```python
from build123d import *

# Parameters (mm, degrees)
BOSS_EXTRUDE1_DEPTH          = 45
SKETCH2_W                    = 42
SKETCH2_H                    = 46.212418486
CUT_EXTRUDE1_DEPTH           = 23
SKETCH3_W                    = 39
SKETCH3_H                    = 1.5
BOSS_EXTRUDE2_DEPTH          = 2
SKETCH4_W                    = 39
SKETCH4_H                    = 1.5
BOSS_EXTRUDE3_DEPTH          = 3.5
SKETCH5_W                    = 39
SKETCH5_H                    = 1.5
BOSS_EXTRUDE4_DEPTH          = 2
SKETCH6_W                    = 39
SKETCH6_H                    = 1.5
BOSS_EXTRUDE5_DEPTH          = 3.5
F_8_0_8_DIAMETER_HOLE1_D     = 8
F_8_0_8_DIAMETER_HOLE1_DEPTH = 1.5
F_8_0_8_DIAMETER_HOLE2_D     = 8
F_8_0_8_DIAMETER_HOLE2_DEPTH = 1.5
F_8_0_8_DIAMETER_HOLE3_D     = 8
F_8_0_8_DIAMETER_HOLE3_DEPTH = 1.5
FILLET1_R                    = 1.5
SKETCH13_R                   = 1
CUT_EXTRUDE2_DEPTH           = 2
SKETCH14_W                   = 11
SKETCH14_H                   = 8
CUT_EXTRUDE3_DEPTH           = 45
FILLET2_R                    = 0.5


with BuildPart() as part:
    # Sketch1 → Boss-Extrude1 (new body)
    with BuildSketch(Plane(origin=(22.5, 0, 0), x_dir=(0, 0, -1), z_dir=(1, 0, 0))):
        with BuildLine():
            Line((-11, 30), (-11, 0))
            ThreePointArc((-11, 0), (0, -11), (11, 0))
            Line((11, 0), (11, 30))
            Line((11, 30), (-11, 30))
        make_face()
    extrude(amount=-BOSS_EXTRUDE1_DEPTH)

    # Sketch2 → Cut-Extrude1 (cut, through all)
    with BuildSketch(Plane.XY.offset(11)):
        with Locations((0, 5.393790757)):
            Rectangle(SKETCH2_W, SKETCH2_H)
    extrude(amount=-CUT_EXTRUDE1_DEPTH, mode=Mode.SUBTRACT)

    # Sketch3 → Boss-Extrude2 (add)
    with BuildSketch(Plane(origin=(0, 0, -11), x_dir=(-1, 0, 0), z_dir=(0, 0, -1))):
        with Locations((0, 29.25)):
            Rectangle(SKETCH3_W, SKETCH3_H)
    extrude(amount=BOSS_EXTRUDE2_DEPTH)

    # Sketch4 → Boss-Extrude3 (add)
    with BuildSketch(Plane.XZ.offset(-28.5)):
        with Locations((0, -12.25)):
            Rectangle(SKETCH4_W, SKETCH4_H)
    extrude(amount=BOSS_EXTRUDE3_DEPTH)

    # Sketch5 → Boss-Extrude4 (add)
    with BuildSketch(Plane.XY.offset(11)):
        with Locations((0, 29.25)):
            Rectangle(SKETCH5_W, SKETCH5_H)
    extrude(amount=BOSS_EXTRUDE4_DEPTH)

    # Sketch6 → Boss-Extrude5 (add)
    with BuildSketch(Plane.XZ.offset(-28.5)):
        with Locations((0, 12.25)):
            Rectangle(SKETCH6_W, SKETCH6_H)
    extrude(amount=BOSS_EXTRUDE5_DEPTH)

    # Ø8.0 (8) Diameter Hole1
    with Locations(Plane(origin=(0, 28.5, 0), x_dir=(-1, 0, 0), z_dir=(0, -1, 0))):
        with Locations((0, 0)):
            Hole(F_8_0_8_DIAMETER_HOLE1_D / 2, depth=F_8_0_8_DIAMETER_HOLE1_DEPTH)

    # Ø8.0 (8) Diameter Hole2
    with Locations(Plane(origin=(-21, 0, 0), x_dir=(0, 0, -1), z_dir=(1, 0, 0))):
        with Locations((0, 0)):
            Hole(F_8_0_8_DIAMETER_HOLE2_D / 2, depth=F_8_0_8_DIAMETER_HOLE2_DEPTH)

    # Ø8.0 (8) Diameter Hole3
    with Locations(Plane.ZY.offset(-21)):
        with Locations((0, 0)):
            Hole(F_8_0_8_DIAMETER_HOLE3_D / 2, depth=F_8_0_8_DIAMETER_HOLE3_DEPTH)

    # Fillet1
    fillet1_edges = [part.edges().sort_by_distance(p)[0] for p in [
        (0, 30, -13),
        (-22.5, 30, 0),
        (22.5, 30, 0),
        (0, 30, 13),
    ]]
    fillet(fillet1_edges, radius=FILLET1_R)

    # Sketch13 → Cut-Extrude2 (cut)
    with BuildSketch(Plane(origin=(0, 30, 0), x_dir=(1, 0, 0), z_dir=(0, 1, 0))):
        with Locations((0, 8)):
            Circle(SKETCH13_R)
        with Locations((0, -8)):
            Circle(SKETCH13_R)
    extrude(amount=-CUT_EXTRUDE2_DEPTH, mode=Mode.SUBTRACT)

    # Sketch14 → Cut-Extrude3 (cut)
    with BuildSketch(Plane(origin=(22.5, 0, 0), x_dir=(0, 0, -1), z_dir=(1, 0, 0))):
        with Locations((0, 18)):
            Rectangle(SKETCH14_W, SKETCH14_H)
    extrude(amount=-CUT_EXTRUDE3_DEPTH, mode=Mode.SUBTRACT)

    # Fillet2
    fillet2_edges = [part.edges().sort_by_distance(p)[0] for p in [
        (-21.75, 14, 5.5),
        (21.75, 14, 5.5),
        (-21.75, 22, 5.5),
        (21.75, 22, 5.5),
        (-21.75, 22, -5.5),
        (21.75, 22, -5.5),
        (-21.75, 14, -5.5),
        (21.75, 14, -5.5),
    ]]
    fillet(fillet2_edges, radius=FILLET2_R)


solid = part.part
```
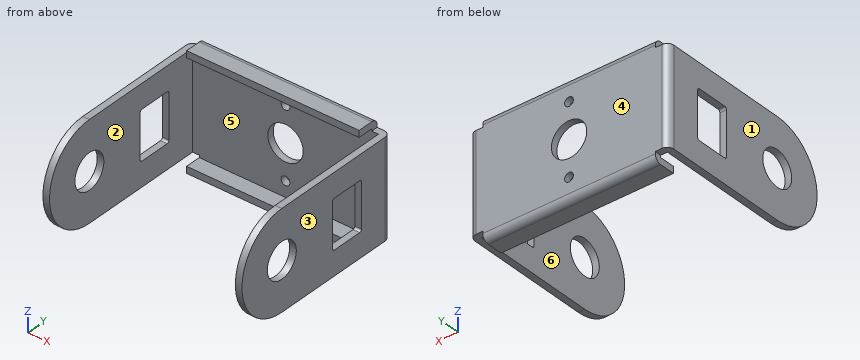
Geometry check sheet. Reference: the model listing, model coordinates, mm. Face numbers are marked on the shaded views. A direction names the side the tool comes from. Give positions to 0.01 mm unless a question says otherwise; leave off trailing zeros. Loops run counter-clockwise (first coordinate to the right, second up) from the corner with the lowest first, then second, coordinate; pieces in that order, holes last. Notation, with made-up numbers: M 88,65 L 96,65 A14 ccw 96,87 Z; hole C 16.5,-27.5 d11. An arc over 180 degrees is marked long. Write item = value, one per line.
(1) Sectioned sample at A-A, the plane y = 10.5. Record the cut outline in (x, z), plus the area to 3 significant figures.
Answer below:
outline = M -22.5,-11 L -21,-11 L -21,11 L -22.5,11 Z; M 21,-11 L 22.5,-11 L 22.5,11 L 21,11 Z
area = 66.0 mm2
(2) Sectioned sample at D-D, the plane y = 3. Record the cut outline in (x, z).
Answer below:
outline = M -22.5,-11 L -21,-11 L -21,-2.65 L -22.5,-2.65 Z; M -22.5,2.65 L -21,2.65 L -21,11 L -22.5,11 Z; M 21,-11 L 22.5,-11 L 22.5,-2.65 L 21,-2.65 Z; M 21,2.65 L 22.5,2.65 L 22.5,11 L 21,11 Z
(3) Sectioned sample at C-C, the plane z = 0. State how many separate pieces and enclosed holes the cut face has, plus the area to 3 significant figures.
Answer below:
separate_pieces = 6
enclosed_holes = 0
area = 125 mm2
(4) Gauge pin test, flat ends, axial feed: pin 1 Ø3.5 at (x, y) = (20.5, 11.5) entering from -Z; pin 2 Ø1.6 at (y, z) = (27, 12.5) entering from +X; pin 3 Ø11.5 at (x, z) = (-10, 4.5) entering from -Y; pin 4 Ø0.9 at (x, y) = (-20.5, 8) entering from -Z. Record the tip position at first contact, or that the pin passes through.
Answer below:
pin_1 = -11
pin_2 = 19.5
pin_3 = 28.5
pin_4 = through
(5) Tool access check on the marked faces 5 and 6. Record the directions out of +Z, -Z, +X, -X, +Y, -Y that give a thin tool (end or side, any length) a straight path to the whole face; none if there is none.
Answer below:
face_5 = -Y
face_6 = +Z, -Z, -Y
(6) Sectioned sample at B-B, the plane x = 0. Record the cut outline in (y, z).
Answer below:
outline = M 25,-13 L 28.5,-13 A1.5 ccw 30,-11.5 L 30,-9 L 28.5,-9 L 28.5,-11.5 L 25,-11.5 Z; M 25,11.5 L 28.5,11.5 L 28.5,9 L 30,9 L 30,11.5 A1.5 ccw 28.5,13 L 25,13 Z; M 28.5,-7 L 30,-7 L 30,-4 L 28.5,-4 Z; M 28.5,4 L 30,4 L 30,7 L 28.5,7 Z
(7) Material ranges on line 1 (X direction, y = 13, z = 3); line 2 (Z direction, x = 0, y = 29.1); line 3 (Z direction, x = 0, y = 29.35), recorded low to high. Write a range as [from, to].
Answer below:
line_1 = [-22.5, -21], [21, 22.5]
line_2 = [-12.87, -9], [-7, -4], [4, 7], [9, 12.87]
line_3 = [-12.74, -9], [-7, -4], [4, 7], [9, 12.74]
(8) Release check for a two-part mould opening along X. For the marked faces 1, 2, 3 and 4 record: released by +X, released by -X, zero draft, split by the parting line, or undercut.
Answer below:
face_1 = released by -X
face_2 = undercut
face_3 = released by +X
face_4 = zero draft
